Geometry: final body of the model. Coordinates: model frame, mm. Face numbers are marked on the shaded views. A direction names the side the tool comes from. Round coordinates to 2 decimals unless told otherwise and drop trailing zeros. Order: outer loops, then holes, each group sorted by start corner. A loop starts at its lowest first (then second) coordinate and runs counter-clockwise, first axis right, second up. Notation, with made-up numbers: (48, 13.25) -> (84, 13.25) arc R14 cw to (84, 24.25) -> close; hole circle Ø7 at (35, 47). An arc over 180 degrees is marked (long way). Put each result on its own line as item: value.
```python
from build123d import *

# Parameters (mm, degrees)
SKETCH_R        = 3
PAD_DEPTH       = 10
SKETCH001_R     = 1
POCKET_DEPTH    = 90.211236
POCKET001_DEPTH = 3
POCKET002_DEPTH = 86.211236


with BuildPart() as part:
    # Sketch → Pad (new body)
    with BuildSketch(Plane.XY):
        with BuildLine():
            ThreePointArc((-27.000023, 7), (-34, 0), (-27.000023, -7))
            Line((-27.000023, -7), (0, -7))
            Line((0, -7), (0, 7))
            Line((-27.000023, 7), (0, 7))
        make_face()
        with Locations((-27, 0)):
            Circle(SKETCH_R, mode=Mode.SUBTRACT)
    pad = extrude(amount=PAD_DEPTH)

    # Sketch001 → Pocket (cut, through all)
    with BuildSketch(Plane.XZ.offset(7)):
        with Locations((-13, 7.5)):
            Circle(SKETCH001_R)
    pocket = extrude(amount=-POCKET_DEPTH, mode=Mode.SUBTRACT)

    # Sketch002 (on Face5 of Pocket) → Pocket001 (cut)
    with BuildSketch(Plane.XY.offset(10)):
        Polygon((-22, 2.886751), (-27, 5.773503), (-32, 2.886751), (-32, -2.886751), (-27, -5.773503), (-22, -2.886751), align=None)
    pocket001 = extrude(amount=-POCKET001_DEPTH, mode=Mode.SUBTRACT)

    # Sketch003 (on Face5 of Pocket001) → Pocket002 (cut, through all)
    with BuildSketch(Plane.XY.offset(10)):
        with BuildLine():
            Line((0, -2), (-18, -2))
            ThreePointArc((-20, -1.6e-05), (-19.414208, -1.414219), (-18, -2))
            ThreePointArc((-20, -1.6e-05), (-22.050255, 4.94975), (-27.000023, 7))
            Line((-27.000023, 7), (0, 7))
            Line((0, -2), (0, 7))
        make_face()
    pocket002 = extrude(amount=-POCKET002_DEPTH, mode=Mode.SUBTRACT)

    # Mirrored: Pad, Pocket, Pocket001, Pocket002 across Sketch003 V_Axis
    add(pad.mirror(Plane(origin=(0, 0, 10), x_dir=(0, 0, 1), z_dir=(1, 0, 0))))
    add(pocket.mirror(Plane(origin=(0, 0, 10), x_dir=(0, 0, 1), z_dir=(1, 0, 0))), mode=Mode.SUBTRACT)
    add(pocket001.mirror(Plane(origin=(0, 0, 10), x_dir=(0, 0, 1), z_dir=(1, 0, 0))), mode=Mode.SUBTRACT)
    add(pocket002.mirror(Plane(origin=(0, 0, 10), x_dir=(0, 0, 1), z_dir=(1, 0, 0))), mode=Mode.SUBTRACT)


solid = part.part
```
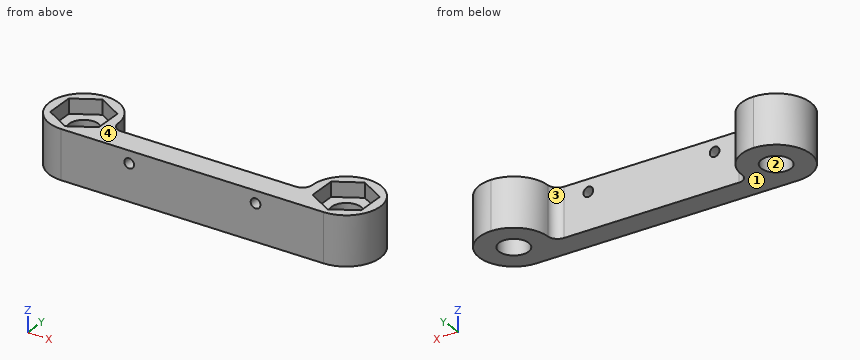
1. Set-up query: the marked faces 3 and 4. Return all of +Z, -Z, +X, -X, +Y, -Y with unobstructed straight access to the full face (end or side cutting, diameter ignored); none if empty.
Ans:
face 3: +Z, -Z, +Y
face 4: +Z, +X, -X, +Y, -Y
2. Cut plane B-B on z = 2. Return loops of the section in (x, y).
Ans:
outline: (-27, -7) -> (27, -7) arc R7 ccw (long way) to (20, 0) arc R2 cw to (18, -2) -> (-18, -2) arc R2 cw to (-20, 0) arc R7 ccw (long way) to start; hole circle Ø6 at (-27, 0); hole circle Ø6 at (27, 0)
3. Contact query for flat-ended pins moving along their axis: P1, Ø2.5, axis at y = 0.5, z = 8.5, coming from the +X side; P2, Ø1.2, axis at x = 13, z = 7.5, coming from the +Y side; P3, Ø3, axis at x = -13, z = 7.5, coming from the +Y side; P4, Ø3, axis at x = -29, y = 2, coming from the +Z side. Output: stop coordinate, or through.
Ans:
P1: x = 34
P2: through
P3: y = -2
P4: z = 7
4. Material intervals for probe 1 along Z at (x, y) = (13, -3.8); probe 2 along Y at (x, z) = (27, 2.5); probe 3 along X at (y, z) = (2.75, 4.25), sorted ascending.
Ans:
probe 1: 0 to 6.5, 8.5 to 10
probe 2: -7 to -3, 3 to 7
probe 3: -33.44 to -28.2, -25.8 to -20.56, 20.56 to 25.8, 28.2 to 33.44
5. Draft query along X for the marked faces 1 and 2. Return one class per face: +X half, -X half, draft (parallel to the pull), parting line (faces both ways), or undercut.
Ans:
face 1: draft
face 2: undercut
6. Cut plane A-A on x = 13. Return loops of the section in (y, z), and give its area (3 significant figures).
Ans:
outline: (-7, 0) -> (-2, 0) -> (-2, 6.5) -> (-7, 6.5) -> close; (-7, 8.5) -> (-2, 8.5) -> (-2, 10) -> (-7, 10) -> close
area: 40.0 mm²
7. Cut plane C-C on y = -4.5. Return loops of the section in (x, z), and give its area (3 significant figures).
Ans:
outline: (-32.36, 0) -> (32.36, 0) -> (32.36, 10) -> (29.21, 10) -> (29.21, 7) -> (24.79, 7) -> (24.79, 10) -> (-24.79, 10) -> (-24.79, 7) -> (-29.21, 7) -> (-29.21, 10) -> (-32.36, 10) -> close; hole circle Ø2 at (-13, 7.5); hole circle Ø2 at (13, 7.5)
area: 614 mm²
8. Cut plane D-D on x = 5. Return loops of the section in (y, z).
Ans:
outline: (-7, 0) -> (-2, 0) -> (-2, 10) -> (-7, 10) -> close
